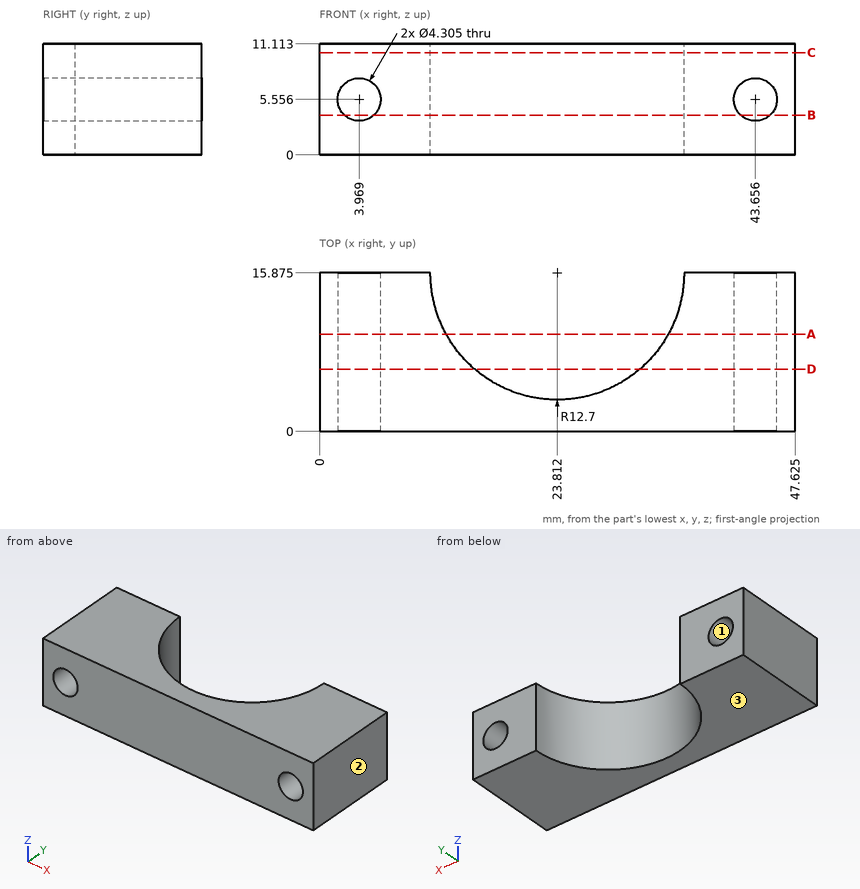
Could you check a few things on this drawing? It's one solid part, dimensions in mm from its lowest x, y, z. Coordinates: 2 decimals unless noted, no trailing zeros. Order: outer loops, then holes, each group sorted by start corner. A loop starts at its lowest first (then second) coordinate and runs counter-clockwise, first axis right, second up. Notation, with made-up numbers: M 38.25,43.5 L 75.25,43.5 A11 ccw 75.25,64.5 Z; hole C 33,35.25 d5. An arc over 180 degrees is marked long. Answer as CSV lines item,"result".
(1) I'm going to push flat-ended pins straight in: pin 1 (1.5 mm diameter, centred on x = 34, z = 4.5, fed in from +Y); pin 2 (1 mm diameter, centred on x = 18, z = 9.5, fed in from +Y) (1 decimal). Where does each tip first touch, or does it pass through?
Geometry check:
pin 1,"y = 9.42"
pin 2,"y = 4.9"
(2) Please list where these lines run through material, in increasing order: L1, parallel to X at y = 1, z = 7.5 (1 decimal); L2, parallel to Z at x = 43.5, y = 11; L3, parallel to X at y = 4.75, z = 7.25 (1 decimal).
Geometry check:
L1,"0 to 3, 4.9 to 42.7, 44.6 to 47.6"
L2,"0 to 3.41, 7.7 to 11.11"
L3,"0 to 2.6, 5.3 to 17.7, 29.9 to 42.3, 45 to 47.6"
(3) Suppose I cut it at A-A on y = 9.75. Please give me the cut outline in (x, z) (1 decimal), plus the area to 3 significant figures.
Geometry check:
outline,"M 0,0 L 12.7,0 L 12.7,11.1 L 0,11.1 Z; M 34.9,0 L 47.6,0 L 47.6,11.1 L 34.9,11.1 Z; hole C 4,5.6 d4.3; hole C 43.7,5.6 d4.3"
area,"253 mm^2"
(4) Suppose I cut it at D-D on y = 6.25. Please give me the cut outline in (x, z) (1 decimal), plus the area to 3 significant figures.
Geometry check:
outline,"M 0,0 L 15.5,0 L 15.5,11.1 L 0,11.1 Z; M 32.1,0 L 47.6,0 L 47.6,11.1 L 32.1,11.1 Z; hole C 4,5.6 d4.3; hole C 43.7,5.6 d4.3"
area,"316 mm^2"
(5) Suppose I cut it at C-C on z = 10.25. Please give me the cut outline in (x, y) (1 decimal), plus the area to 3 significant figures.
Geometry check:
outline,"M 0,0 L 47.6,0 L 47.6,15.9 L 36.5,15.9 A12.7 cw 11.1,15.9 L 0,15.9 Z"
area,"503 mm^2"
(6) If we mould it in two halves opening along Z, with no side actions, what happens to the marked faces 1, 2 and 3? For each: released by +Z, released by -Z, zero draft, split by the parting line, or undercut.
Geometry check:
face 1,"undercut"
face 2,"zero draft"
face 3,"released by -Z"
(7) Suppose I cut it at B-B on z = 4. Please give me the cut outline in (x, y) (1 decimal).
Geometry check:
outline,"M 0,0 L 2.5,0 L 2.5,15.9 L 0,15.9 Z; M 5.5,0 L 42.2,0 L 42.2,15.9 L 36.5,15.9 A12.7 cw 11.1,15.9 L 5.5,15.9 Z; M 45.1,0 L 47.6,0 L 47.6,15.9 L 45.1,15.9 Z"
